Build history of the part. All positions in model axes, mm. Face numbers are marked on the shaded views. A direction names the side the tool comes from. Round coordinates to 2 decimals unless told otherwise and drop trailing zeros. Write each loop counter-clockwise with the first axis right and the second up, starting at its lowest first coordinate (ties: lowest second). Pieces come first, ordered by that corner, then holes. Notation, with made-up numbers: M 75,-37.75 L 88,-37.75 A25 cw 88,-22.75 Z; hole C 68,25.5 d9. An arc over 180 degrees is marked long. Use a Markdown table: item, result.
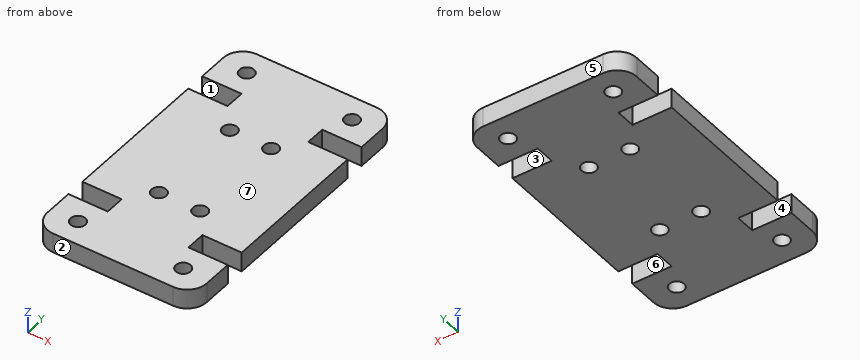
from build123d import *

# Parameters (mm, degrees)
SKETCH1_R           = 0.75
BOSS_EXTRUDE1_DEPTH = 2


with BuildPart() as part:
    # Sketch1 → Boss-Extrude1 (new body)
    with BuildSketch(Plane.XY):
        with BuildLine():
            Line((0, 22.14), (0, 7))
            Line((0, 7), (4, 7))
            Line((4, 7), (4, 5))
            Line((4, 5), (0, 5))
            Line((0, 5), (0, 2))
            ThreePointArc((0, 2), (0.585786438, 0.585786438), (2, 0))
            Line((2, 0), (14.2, 0))
            ThreePointArc((14.2, 0), (15.614213562, 0.585786438), (16.2, 2))
            Line((16.2, 2), (16.2, 5))
            Line((16.2, 5), (12.2, 5))
            Line((12.2, 5), (12.2, 7))
            Line((12.2, 7), (16.2, 7))
            Line((16.2, 7), (16.2, 22.14))
            Line((16.2, 22.14), (12.2, 22.14))
            Line((12.2, 22.14), (12.2, 24.14))
            Line((12.2, 24.14), (16.2, 24.14))
            Line((16.2, 24.14), (16.2, 27.14))
            ThreePointArc((16.2, 27.14), (15.614213562, 28.554213562), (14.2, 29.14))
            Line((14.2, 29.14), (2, 29.14))
            ThreePointArc((2, 29.14), (0.585786438, 28.554213562), (0, 27.14))
            Line((0, 27.14), (0, 24.14))
            Line((0, 24.14), (4, 24.14))
            Line((4, 24.14), (4, 22.14))
            Line((4, 22.14), (0, 22.14))
        make_face()
        with Locations((13.45, 2.5)):
            Circle(SKETCH1_R, mode=Mode.SUBTRACT)
        with Locations((10.2, 9.5)):
            Circle(SKETCH1_R, mode=Mode.SUBTRACT)
        with Locations((2.75, 26.64)):
            Circle(SKETCH1_R, mode=Mode.SUBTRACT)
        with Locations((6, 19.64)):
            Circle(SKETCH1_R, mode=Mode.SUBTRACT)
        with Locations((6, 9.5)):
            Circle(SKETCH1_R, mode=Mode.SUBTRACT)
        with Locations((2.75, 2.5)):
            Circle(SKETCH1_R, mode=Mode.SUBTRACT)
        with Locations((10.2, 19.64)):
            Circle(SKETCH1_R, mode=Mode.SUBTRACT)
        with Locations((13.45, 26.64)):
            Circle(SKETCH1_R, mode=Mode.SUBTRACT)
    extrude(amount=BOSS_EXTRUDE1_DEPTH)


solid = part.part
Q1. Two-plate mould, pull along Y, no slides. Class the marked faces 4, 5, 6 and 7: +Y half, -Y half, draft (parallel to the pull), parting line (faces both ways), or undercut.
Response values:
| item | result |
|---|---|
| face 4 | undercut |
| face 5 | +Y half |
| face 6 | undercut |
| face 7 | draft |
Q2. Cut at C-C on z = 0.45. Count the separate pieces of the cut face and the enclosed holes in it, and give its area (3 significant figures).
Response values:
| item | result |
|---|---|
| separate pieces | 1 |
| enclosed holes | 8 |
| area | 422 mm2 |
Q3. Which spindle directions (+Z, -Z, +X, -X, +Y, -Y) get a long thin tool onto all of the face, cutting with end or side? Do the marked faces 1, 2 and 3. Say none if no direction does.
Response values:
| item | result |
|---|---|
| face 1 | +Z, -Z, -X |
| face 2 | +Z, -Z, +X, -X, -Y |
| face 3 | +Z, -Z, +X |
Q4. Drill centre lines: L1, parallel to Y at x = 13.45, z = 1.3; L2, parallel to Y at x = 3.75, z = 0.85; L3, parallel to Y at x = 6, z = 0.6. Where is each one in solid material? Low to high.
Response values:
| item | result |
|---|---|
| L1 | y = 0 to 1.75, 3.25 to 5, 7 to 22.14, 24.14 to 25.89, 27.39 to 29.14 |
| L2 | y = 0 to 5, 7 to 22.14, 24.14 to 29.14 |
| L3 | y = 0 to 8.75, 10.25 to 18.89, 20.39 to 29.14 |
Q5. Cut at A-A on x = 2.75. Give the cut face in (y, z), and give its area (3 significant figures).
Response values:
| item | result |
|---|---|
| outline | M 0,0 L 1.75,0 L 1.75,2 L 0,2 Z; M 3.25,0 L 5,0 L 5,2 L 3.25,2 Z; M 7,0 L 22.14,0 L 22.14,2 L 7,2 Z; M 24.14,0 L 25.89,0 L 25.89,2 L 24.14,2 Z; M 27.39,0 L 29.14,0 L 29.14,2 L 27.39,2 Z |
| area | 44.3 mm2 |
Q6. Cut at D-D on x = 10.2. Give the cut face in (y, z).
Response values:
| item | result |
|---|---|
| outline | M 0,0 L 8.75,0 L 8.75,2 L 0,2 Z; M 10.25,0 L 18.89,0 L 18.89,2 L 10.25,2 Z; M 20.39,0 L 29.14,0 L 29.14,2 L 20.39,2 Z |
Q7. Cut at B-B on y = 9.5. Give the cut face in (x, z), and give its area (3 significant figures).
Response values:
| item | result |
|---|---|
| outline | M 0,0 L 5.25,0 L 5.25,2 L 0,2 Z; M 6.75,0 L 9.45,0 L 9.45,2 L 6.75,2 Z; M 10.95,0 L 16.2,0 L 16.2,2 L 10.95,2 Z |
| area | 26.4 mm2 |
Q8. Drop flat-ended pins along their axis: P1, Ø1.2, axis at x = 6, y = 9.5, coming from the -Z side; P2, Ø1, axis at x = 15, z = 1.5, coming from the -Y side. Give the stop position or say it passes through.
Response values:
| item | result |
|---|---|
| P1 | passes through |
| P2 | stops at y = 0.02 |
